Can you work these out from the model? Positions are in its coordinate system, mm. A direction names the side the tool comes from. Round coordinates to 2 decimals unless told otherwise and drop trailing zeros. Order: outer loops, then holes, each group sorted by start corner. A loop starts at its lowest first (then second) coordinate and runs counter-clockwise, first axis right, second up. Notation, with made-up numbers: (78, 35) - (136, 35) arc R16 cw to (136, 53) - close; hole circle Ø5 at (-2.5, 57). An arc over 180 degrees is marked (long way). Write item = value, one per line.
from build123d import *

# Parameters (mm, degrees)
SKETCH_W        = 9.5
SKETCH_H        = 11.35
PAD_DEPTH       = 1
POCKET002_DEPTH = 0.5
POCKET003_DEPTH = 0.5


with BuildPart() as part:
    # Sketch → Pad (new body)
    with BuildSketch(Plane.XY):
        with Locations((0, -0.825)):
            Rectangle(SKETCH_W, SKETCH_H)
    extrude(amount=PAD_DEPTH)

    # Sketch005 → Pocket002 (cut)
    with BuildSketch(Plane.XY):
        with BuildLine():
            Line((2.75, 4.85), (4.75, 4.85))
            Line((4.75, 4.85), (4.75, 2.85))
            Line((4.75, 2.85), (3.75, 2.85))
            ThreePointArc((2.75, 3.85), (3.042893, 3.142893), (3.75, 2.85))
            Line((2.75, 3.85), (2.75, 4.85))
        make_face()
    extrude(amount=POCKET002_DEPTH, mode=Mode.SUBTRACT)

    # Sketch006 → Pocket003 (cut)
    with BuildSketch(Plane.XY):
        with BuildLine():
            Line((-4.75, -2.5), (-4.75, -4.5))
            Line((-4.75, -4.5), (-3.75, -4.5))
            ThreePointArc((-3.75, -4.5), (-2.75, -3.5), (-3.75, -2.5))
            Line((-4.75, -2.5), (-3.75, -2.5))
        make_face()
    extrude(amount=POCKET003_DEPTH, mode=Mode.SUBTRACT)


solid = part.part
(1) If we section it at B-B (y = -3.5): Write out the boundary of the cut face in (x, z), plus the area to 3 significant figures.
Computed:
outline = (-4.75, 0.5) - (-2.75, 0.5) - (-2.75, 0) - (4.75, 0) - (4.75, 1) - (-4.75, 1) - close
area = 8.50 mm^2
(2) Will this pin go through, and if not, where does the flat tip stop? P1, Ø1.6, axis at x = 4, y = 3.5, coming from the -Z side.
Computed:
P1 = 0
(3) Thinking about a two-plate mould opening in Y: for faces 1 (the face through (-0.1, 4.85, 0.5)), 2 (the face through (-4, -3, 0.5)), 3 (the face through (0, -1, 0)), which applies, +Y half, -Y half, draft (parallel to the pull), parting line (faces both ways), or undercut?
Computed:
face_1 = +Y half
face_2 = undercut
face_3 = draft
(4) If we section it at A-A (z = 0.35): Write out the boundary of the cut face in (x, y), plus the area to 3 significant figures.
Computed:
outline = (-4.75, -6.5) - (4.75, -6.5) - (4.75, 2.85) - (3.75, 2.85) arc R1 cw to (2.75, 3.85) - (2.75, 4.85) - (-4.75, 4.85) - (-4.75, -2.5) - (-3.75, -2.5) arc R1 cw to (-3.75, -4.5) - (-4.75, -4.5) - close
area = 100 mm^2
(5) If I drill on line 1 (Y direction, x = 4, z = 0.3); line 2 (X direction, y = 4, z = 0.2); line 3 (Y direction, x = -3.5, z = 0.15), over which ranges is the centre line in solid material (lowest first)? Write a range as from..to.
Computed:
line_1 = -6.5..2.85
line_2 = -4.75..2.75
line_3 = -6.5..-4.47, -2.53..4.85
(6) On a 3-axis mill with a long thin cutter (end or side, diameter ignored), from which of +Z, -Z, +X, -X, +Y, -Y can I reach the whole of each face in a straight line? I mean faces 4 (the face through (-2.75, -3.52, 0.25)), 5 (the face through (-0.1, -6.5, 0.5)), 6 (the face through (4, 4, 0.5)). Say none if no direction works.
Computed:
face_4 = -Z, -X
face_5 = +Z, -Z, +X, -X, -Y
face_6 = -Z, +X, +Y
